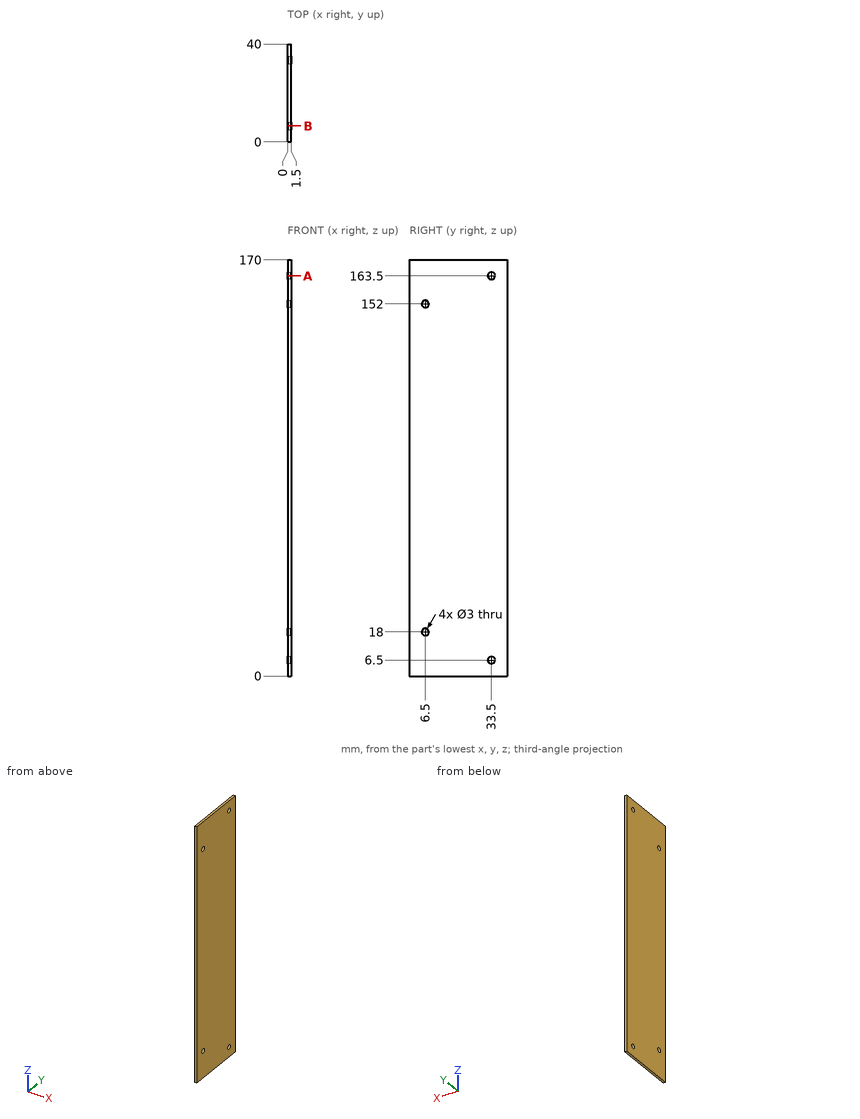
Design review of the part shown in the three views and the two pictorial views. Dimensions are in mm from the part's minimum x, y and z. Coordinates: 2 decimals unless noted, no trailing zeros. Write each loop counter-clockwise with the first axis right and the second up, starting at its lowest first coordinate (ties: lowest second). Pieces come first, ordered by that corner, then holes.
(1) For pin 1 Ø5 at (y, z) = (6.5, 18) entering from +X, flat-tipped, find the tip position at first contact; note if it passes through.
(2) Wall thickness on probe 1 along Y at (x, z) = (1.05, 6.5); probe 2 along Y at (x, z) = (1, 152): over which ranges is each line inside the solid? List them lowest first.
(3) Add section A-A on z = 163.5. Give the boundary of the cut face in (x, y), then the cut area to 3 significant figures.
(4) Add section B-B on y = 6.5. Give the boundary of the cut face in (x, z).
Answer sheet:
1. pin 1: stops at x = 1.5
2. probe 1: y = 0 to 32, 35 to 40
2. probe 2: y = 0 to 5, 8 to 40
3. outline: (0, 0) - (1.5, 0) - (1.5, 32) - (0, 32) - close; (0, 35) - (1.5, 35) - (1.5, 40) - (0, 40) - close
3. area: 55.5 mm2
4. outline: (0, 0) - (1.5, 0) - (1.5, 16.5) - (0, 16.5) - close; (0, 19.5) - (1.5, 19.5) - (1.5, 150.5) - (0, 150.5) - close; (0, 153.5) - (1.5, 153.5) - (1.5, 170) - (0, 170) - close
